```python
from build123d import *

# Parameters (mm, degrees)
F0_R     = 2
F1_DEPTH = 5
F2_DEPTH = 2


with BuildPart() as f1:
    # F0 (on Top) → F1 (new body)
    with BuildSketch(Plane.XY):
        with BuildLine():
            ThreePointArc((2.645751, -3), (3.645751, -1.645751), (4, 0))
            ThreePointArc((4, 0), (3.645751, 1.645751), (2.645751, 3))
            ThreePointArc((2.645751, 3), (1.414214, 3.741657), (0, 4))
            ThreePointArc((0, 4), (-4, 0), (0, -4))
            ThreePointArc((0, -4), (1.414214, -3.741657), (2.645751, -3))
        make_face()
        Circle(F0_R, mode=Mode.SUBTRACT)
        with BuildLine():
            ThreePointArc((0, 4), (1.414214, 3.741657), (2.645751, 3))
            Line((2.645751, 3), (26.664249, 3))
            ThreePointArc((26.664249, 3), (27.895786, 3.741657), (29.31, 4))
            Line((29.31, 4), (0, 4))
        make_face()
        with BuildLine():
            Line((26.664249, -3), (2.645751, -3))
            ThreePointArc((2.645751, -3), (1.414214, -3.741657), (0, -4))
            Line((0, -4), (29.31, -4))
            ThreePointArc((29.31, -4), (27.895786, -3.741657), (26.664249, -3))
        make_face()
        with BuildLine():
            ThreePointArc((29.31, 4), (27.895786, 3.741657), (26.664249, 3))
            ThreePointArc((26.664249, 3), (25.31, 0), (26.664249, -3))
            ThreePointArc((26.664249, -3), (27.895786, -3.741657), (29.31, -4))
            ThreePointArc((29.31, -4), (32.138427, -2.828427), (33.31, 0))
            ThreePointArc((33.31, 0), (32.138427, 2.828427), (29.31, 4))
        make_face()
        with Locations((29.31, 0)):
            Circle(F0_R, mode=Mode.SUBTRACT)
    extrude(amount=F1_DEPTH)

    # F0 (on Top) → F2 (join)
    with BuildSketch(Plane.XY):
        with BuildLine():
            ThreePointArc((2.645751, -3), (3.645751, -1.645751), (4, 0))
            ThreePointArc((4, 0), (3.645751, 1.645751), (2.645751, 3))
            ThreePointArc((2.645751, 3), (1.414214, 3.741657), (0, 4))
            ThreePointArc((0, 4), (-4, 0), (0, -4))
            ThreePointArc((0, -4), (1.414214, -3.741657), (2.645751, -3))
        make_face()
        Circle(F0_R, mode=Mode.SUBTRACT)
        with BuildLine():
            ThreePointArc((0, 4), (1.414214, 3.741657), (2.645751, 3))
            Line((2.645751, 3), (26.664249, 3))
            ThreePointArc((26.664249, 3), (27.895786, 3.741657), (29.31, 4))
            Line((29.31, 4), (0, 4))
        make_face()
        with BuildLine():
            Line((26.664249, -3), (2.645751, -3))
            ThreePointArc((2.645751, -3), (1.414214, -3.741657), (0, -4))
            Line((0, -4), (29.31, -4))
            ThreePointArc((29.31, -4), (27.895786, -3.741657), (26.664249, -3))
        make_face()
        with BuildLine():
            ThreePointArc((29.31, 4), (27.895786, 3.741657), (26.664249, 3))
            ThreePointArc((26.664249, 3), (25.31, 0), (26.664249, -3))
            ThreePointArc((26.664249, -3), (27.895786, -3.741657), (29.31, -4))
            ThreePointArc((29.31, -4), (32.138427, -2.828427), (33.31, 0))
            ThreePointArc((33.31, 0), (32.138427, 2.828427), (29.31, 4))
        make_face()
        with Locations((29.31, 0)):
            Circle(F0_R, mode=Mode.SUBTRACT)
        with BuildLine():
            ThreePointArc((2.645751, 3), (3.645751, 1.645751), (4, 0))
            ThreePointArc((4, 0), (3.645751, -1.645751), (2.645751, -3))
            Line((2.645751, -3), (26.664249, -3))
            ThreePointArc((26.664249, -3), (25.31, 0), (26.664249, 3))
            Line((26.664249, 3), (2.645751, 3))
        make_face()
    extrude(amount=F2_DEPTH)


solid = f1.part
```
Can you work these out from the model? Positions are in its coordinate system, mm. A direction names the side the tool comes from. Give positions to 0.01 mm unless a question says otherwise; leave off trailing zeros. Write each loop counter-clockwise with the first axis right and the second up, starting at its lowest first coordinate (ties: lowest second). Pieces come first, ordered by that corner, then holes. Notation, with made-up numbers: (29.5, 65) - (59.5, 65) arc R21 ccw to (59.5, 84) - close; hole circle Ø7 at (38.25, -14.5). An arc over 180 degrees is marked (long way). Write item = value, one per line. Start each with the question number.
1. Imagine slicing it at C-C (x = 15). Please give me the cut outline in (y, z).
2. Imagine slicing it at A-A (z = 2.75). Please give me the cut outline in (x, y), and give its area (3 significant figures).
3. On a 3-axis mill with a long thin cutter (end or side, diameter ignored), from which of +Z, -Z, +X, -X, +Y, -Y can I reach the whole of each face in a straight line? I mean faces 4 (the face through (14, 3, 3)), 5 (the face through (15, 4, 2)). Say none if no direction works.
4. Imagine slicing it at D-D (y = 1.25). Please give me the cut outline in (x, z).
5. Thinking about a two-plate mould opening in X: for faces 1 (the face through (0, -2, 2)), 2 (the face through (14, 0, 0)), 3 (the face through (-4, 0, 2)), which applies, released by +X, released by -X, zero draft, split by the parting line, or undercut?
6. Imagine slicing it at B-B (z = 0.4). Please give me the cut outline in (x, y).
7. Please list where these lines run through material, in increasing order: line 1 (Y direction, x = 17.5, z = 3.45); line 2 (Y direction, x = 29.31, z = 1.4); line 3 (X direction, y = 0.25, z = 4.35).
8. For pin 1 (1 mm diameter, centred on y = -1, z = 3.5, fed in from +X); pin 2 (1 mm diameter, centred on x = 11.5, y = 1, fed in from -Z), each with a flat end and sliding along its axis, tell me the tip position at first contact or that it passes through.
Worked answers:
q1.outline = (-4, 0) - (4, 0) - (4, 5) - (3, 5) - (3, 2) - (-3, 2) - (-3, 5) - (-4, 5) - close
q2.outline = (0, -4) - (29.31, -4) arc R4 ccw to (29.31, 4) - (0, 4) arc R4 ccw to start; hole circle Ø4 at (0, 0); hole (2.65, -3) - (26.66, -3) arc R4 cw to (26.66, 3) - (2.65, 3) arc R4 cw to (4, 0) arc R4 cw to start; hole circle Ø4 at (29.31, 0)
q2.area = 127 mm2
q3.face_4 = +Z
q3.face_5 = +Z, -Z, +X, -X, +Y
q4.outline = (-3.8, 0) - (-1.56, 0) - (-1.56, 5) - (-3.8, 5) - close; (1.56, 0) - (27.75, 0) - (27.75, 5) - (25.51, 5) - (25.51, 2) - (3.8, 2) - (3.8, 5) - (1.56, 5) - close; (30.87, 0) - (33.11, 0) - (33.11, 5) - (30.87, 5) - close
q5.face_1 = undercut
q5.face_2 = zero draft
q5.face_3 = released by -X
q6.outline = (0, -4) - (29.31, -4) arc R4 ccw to (29.31, 4) - (0, 4) arc R4 ccw to start; hole circle Ø4 at (0, 0); hole circle Ø4 at (29.31, 0)
q7.line_1 = -4 to -3, 3 to 4
q7.line_2 = -4 to -2, 2 to 4
q7.line_3 = -3.99 to -1.98, 1.98 to 3.99, 25.32 to 27.33, 31.29 to 33.3
q8.pin_1 = 33.28
q8.pin_2 = 0
